Source: CAD feature listing. Evaluate the final solid. Frame: model axes, mm. Face numbers are marked on the shaded views. A direction names the side the tool comes from. Round coordinates to 2 decimals unless told otherwise and drop trailing zeros. Write each loop counter-clockwise with the first axis right and the second up, starting at its lowest first coordinate (ties: lowest second). Pieces come first, ordered by that corner, then holes.
```python
from build123d import *

# Parameters (mm, degrees)
F1_DEPTH  = 2
F0_W      = 2
F0_H      = 35
F2_DEPTH  = 10
F0_W_2    = 4
F0_H_2    = 5
F3_DEPTH  = 7
F4_W      = 4
F4_H      = 3.5
F5_DEPTH  = 5
F6_R      = 1.5
F7_DEPTH  = 2
F8_DEPTH  = 5
F9_DEPTH  = 5
F10_DEPTH = 5


with BuildPart() as f1:
    # F0 (on Top) → F1 (new body)
    with BuildSketch(Plane.XY):
        Polygon((11.5, 17.5), (-11.5, 17.5), (-11.5, -17.5), (-2, -17.5), (2, -17.5), (11.5, -17.5), align=None)
    extrude(amount=F1_DEPTH)

    # F0 (on Top) → F2 (join)
    with BuildSketch(Plane.XY):
        with Locations((-12.5, 0)):
            Rectangle(F0_W, F0_H)
        with Locations((12.5, 0)):
            Rectangle(F0_W, F0_H)
    extrude(amount=F2_DEPTH)

    # F0 (on Top) → F3 (join)
    with BuildSketch(Plane.XY):
        with Locations((0, -20)):
            Rectangle(F0_W_2, F0_H_2)
    extrude(amount=F3_DEPTH)

    # F4 (on face) → F5 (join)
    with BuildSketch(Plane(origin=(0, -17.5, 0), x_dir=(-1, 0, 0), z_dir=(0, 1, 0))):
        with Locations((0, 5.25)):
            Rectangle(F4_W, F4_H)
    extrude(amount=F5_DEPTH)

    # F6
    f6_edges = [f1.edges().sort_by_distance(p)[0] for p in [
        (0, -12.5, 3.5),
    ]]
    fillet(f6_edges, radius=F6_R)

    # F7 (cut): a face of the model
    f7_faces = [f1.faces().sort_by_distance(p)[0] for p in [
        (0, -17.5, 2.75),
    ]]
    extrude(f7_faces, amount=-F7_DEPTH, mode=Mode.SUBTRACT)

    # F8 (cut): a face of the model
    f8_faces = [f1.faces().sort_by_distance(p)[0] for p in [
        (0, 17.5, 0.287923601),
    ]]
    extrude(f8_faces, amount=-F8_DEPTH, mode=Mode.SUBTRACT)

    # F9 (add): faces of the model
    f9_faces = [f1.faces().sort_by_distance(p)[0] for p in [
        (6.75, -17.5, 1.8476024935),
        (-6.75, -17.5, 1.8476024935),
    ]]
    extrude(f9_faces, amount=F9_DEPTH)

    # F10 (cut): a face of the model
    f10_faces = [f1.faces().sort_by_distance(p)[0] for p in [
        (0, 12.5, 0.287923601),
    ]]
    extrude(f10_faces, amount=-F10_DEPTH, mode=Mode.SUBTRACT)


solid = f1.part
```
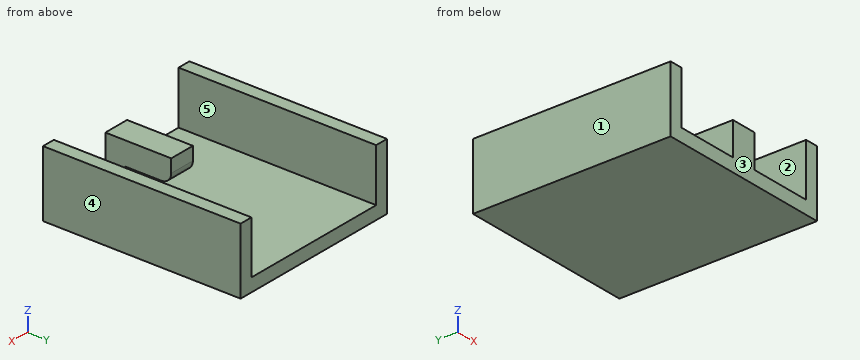
Q1. Mould query, pull axis X, two halves, no side actions, for the marked faces 3, 4 and 5. Classes: pulls with the +X half, pulls with the -X half, needs draft (parallel to the pull), parting line crosses it, or undercut.
Q2. Section query C-C, the plane z = 8.25. Output: boundary loops of the cut face in (x, y), and give its area (3 significant figures).
Q3. Section query D-D, the plane x = -0.25. Output: boundary loops of the cut face in (y, z).
Q4. Section query A-A, the plane z = 6.25. Output: boundary loops of the cut face in (x, y).
Q5. Section query B-B, the plane y = -15.5. Output: boundary loops of the cut face in (x, z), and give its area (3 significant figures).
Q6. Pin query (flat end, axial travel): P1, Ø3, axis at x = 0.5, y = -2, coming from the +Z side; P2, Ø1.6, axis at x = 0, z = 3, coming from the +Y side; P3, Ø2, axis at x = 0, z = 6, coming from the +Y side. Return the tip coordinate at first contact, or that it passes through.
Q7. Line query: line 1 (X direction, y = 0, z = 4.25); line 2 (Z direction, x = -9.5, y = -11.75); line 3 (Y direction, x = 0.5, z = 3.25). Output: solid intervals per line, ascending.
Q8. Set-up query: the marked faces 1 and 2. Return all of +Z, -Z, +X, -X, +Y, -Y with unobstructed straight access to the full face (end or side cutting, diameter ignored); none if empty.
Filled in:
1. face 3: needs draft
1. face 4: pulls with the +X half
1. face 5: undercut
2. outline: (-13.5, -22.5) - (-11.5, -22.5) - (-11.5, 7.5) - (-13.5, 7.5) - close; (11.5, -22.5) - (13.5, -22.5) - (13.5, 7.5) - (11.5, 7.5) - close
2. area: 120 mm2
3. outline: (-22.5, 0) - (7.5, 0) - (7.5, 2) - (-19.5, 2) - (-19.5, 3.5) - (-14, 3.5) arc R1.5 ccw to (-12.5, 5) - (-12.5, 7) - (-22.5, 7) - close
4. outline: (-13.5, -22.5) - (-11.5, -22.5) - (-11.5, 7.5) - (-13.5, 7.5) - close; (-2, -22.5) - (2, -22.5) - (2, -12.5) - (-2, -12.5) - close; (11.5, -22.5) - (13.5, -22.5) - (13.5, 7.5) - (11.5, 7.5) - close
5. outline: (-13.5, 0) - (13.5, 0) - (13.5, 10) - (11.5, 10) - (11.5, 2) - (-11.5, 2) - (-11.5, 10) - (-13.5, 10) - close; (-2, 3.5) - (2, 3.5) - (2, 7) - (-2, 7) - close
5. area: 100 mm2
6. P1: stops at z = 2
6. P2: stops at y = -13.1
6. P3: stops at y = -12.5
7. line 1: x = -13.5 to -11.5, 11.5 to 13.5
7. line 2: z = 0 to 2
7. line 3: y = -22.5 to -19.5
8. face 1: +Z, -Z, -X, +Y, -Y
8. face 2: +Z, +Y, -Y
